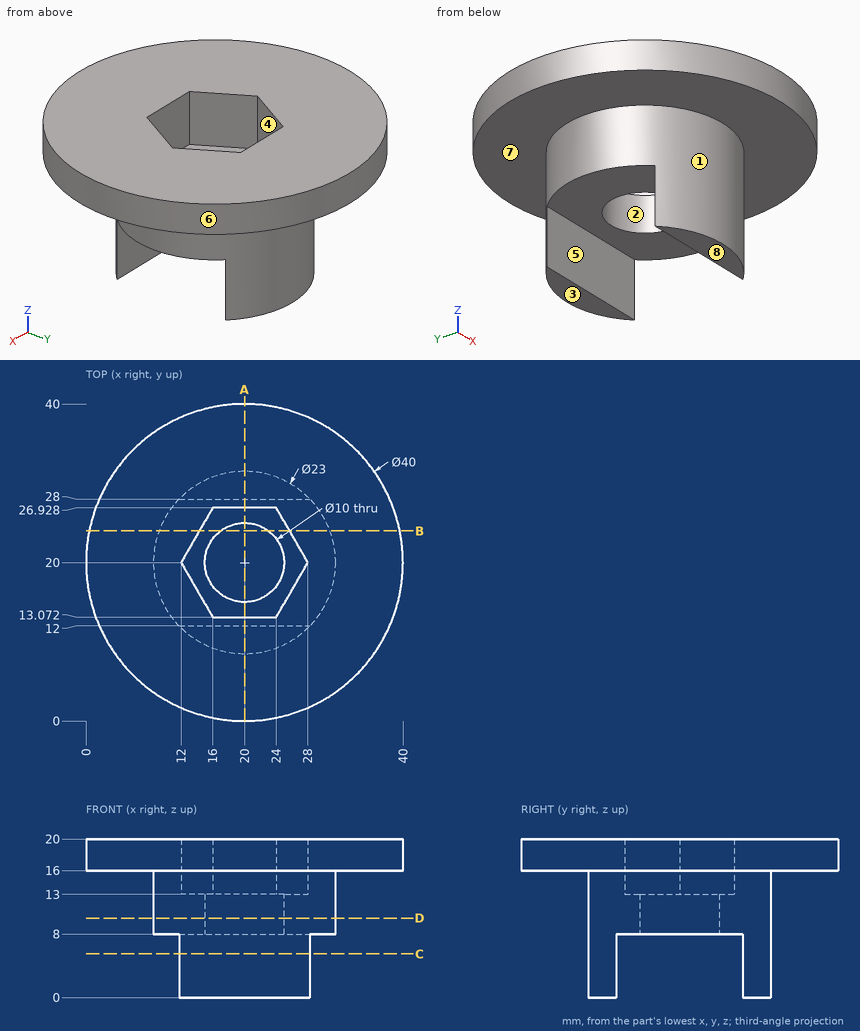
Verification items for this drawing (mm, ordinates from the low corner). A direction names the side the tool comes from. Coordinates: 2 decimals unless noted, no trailing zeros. Order: outer loops, then holes, each group sorted by start corner. A loop starts at its lowest first (then second) coordinate and runs counter-clockwise, first axis right, second up. Notation, with made-up numbers: M 0,-25 L 12,-25 A31 cw 12,14 Z; hole C -14.5,61.5 d7. An arc over 180 degrees is marked long. One line per item, written item: value. Start each with the question number.
Item 1: Thickness scan on probe 1 along Y at (x, z) = (20, 10.4); probe 2 along Z at (x, y) = (10, 4). Record the ranges inside material, lowest first.
Item 2: Access from +Z, -Z, +X, -X, +Y, -Y to the whole of each face (thin tool, end or side, straight path). Record for the marked faces 4, 5, 6, 7 and 8.
Item 3: Sectioned sample at D-D on z = 10. Record the cut outline in (x, y), then the cut area to 3 significant figures.
Item 4: Mould release check, pull along Y, two halves, no side actions. Record for the marked faces 1, 2 and 3: pulls with the +Y half, pulls with the -Y half, needs draft (parallel to the pull), parting line crosses it, or undercut.
Item 5: Sectioned sample at C-C on z = 5.5. Record the cut outline in (x, y), then the cut area to 3 significant figures.
Item 6: Sectioned sample at A-A on x = 20. Record the cut outline in (y, z), then the cut area to 3 significant figures.
Item 7: Sectioned sample at B-B on y = 24. Record the cut outline in (x, z).
Item 8: Depth check by flat-ended pin: P1, Ø6.5, axis at x = 23.5, z = 3.5, coming from the -Y side; P2, Ø1.5, axis at x = 27, z = 11.5, coming from the +Y side; P3, Ø3, axis at x = 25.5, z = 9.5, coming from the +Y side. Enter the tip coordinate at first touch or a pass-through.
Calculated:
1. probe 1: 8.5 to 15, 25 to 31.5
1. probe 2: 16 to 20
2. face 4: +Z
2. face 5: -Z, +X, -X
2. face 6: +Z, -Z
2. face 7: -Z
2. face 8: -Z, +X, -X, +Y, -Y
3. outline: C 20,20 d23; hole C 20,20 d10
3. area: 337 mm^2
4. face 1: parting line crosses it
4. face 2: undercut
4. face 3: needs draft
5. outline: M 11.74,12 A11.5 ccw 28.26,12 Z; M 11.74,28 L 28.26,28 A11.5 ccw Z
5. area: 79.8 mm^2
6. outline: M 0,16 L 8.5,16 L 8.5,0 L 12,0 L 12,8 L 15,8 L 15,13 L 13.07,13 L 13.07,20 L 0,20 Z; M 25,8 L 28,8 L 28,0 L 31.5,0 L 31.5,16 L 40,16 L 40,20 L 26.93,20 L 26.93,13 L 25,13 Z
6. area: 253 mm^2
7. outline: M 0.4,16 L 9.22,16 L 9.22,8 L 17,8 L 17,13 L 14.31,13 L 14.31,20 L 0.4,20 Z; M 23,8 L 30.78,8 L 30.78,16 L 39.6,16 L 39.6,20 L 25.69,20 L 25.69,13 L 23,13 Z
8. P1: y = 8.5
8. P2: y = 29.65
8. P3: y = 30.78
